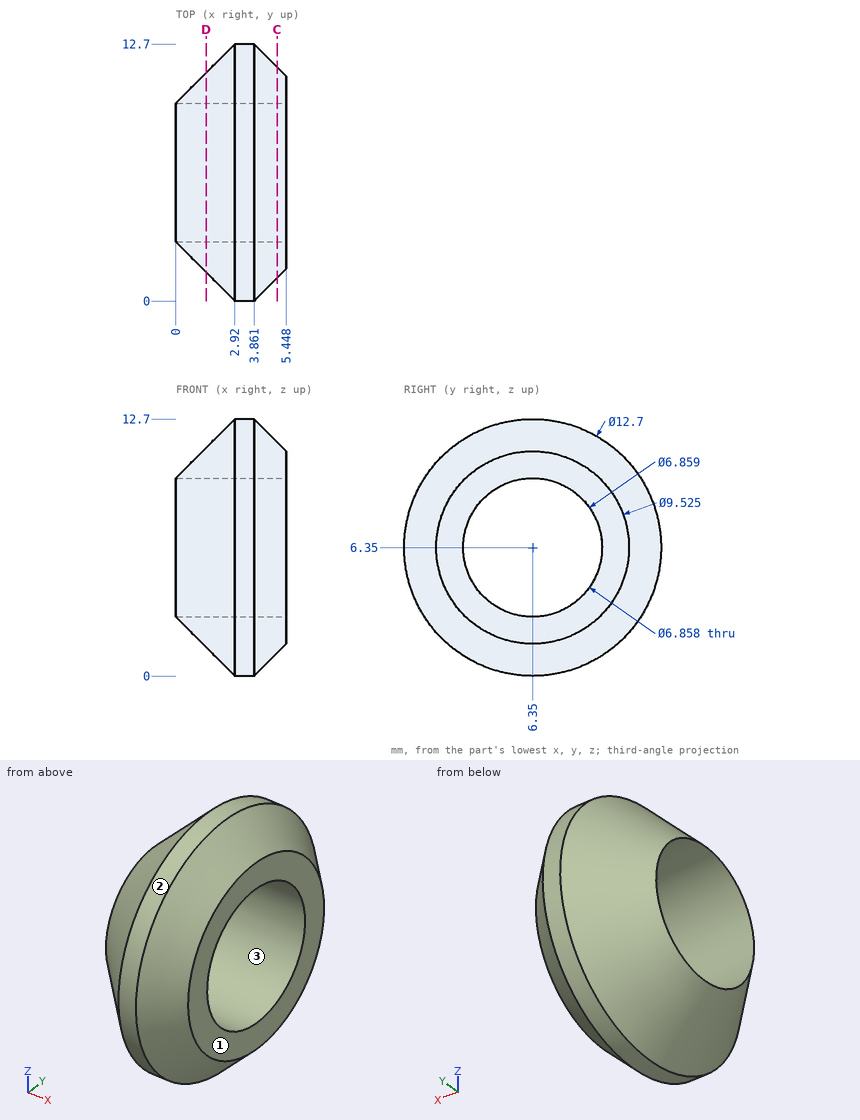
Answer from the drawing. Dimensions are ordinates in mm from the lowest x, y and z of the part. Give positions to 0.01 mm unless a question says otherwise; leave off trailing zeros. Loops run counter-clockwise (first coordinate to the right, second up) from the corner with the lowest first, then second, coordinate; pieces in that order, holes last.
Item 1: The part is cut by section D-D (x = 1.5). Write down the section's boundary in (y, z).
Item 2: Each of these flat-tipped pins is pushed along its axis until it touches: pin 1 Ø1.5 at (x, y) = (1, 2) entering from -Z (1 decimal); pin 2 Ø3 at (x, z) = (2.5, 10.5) entering from -Y; pin 3 Ø1.5 at (y, z) = (8.5, 2.5) entering from -X. Where does it stop, or does it pass through?
Item 3: The part is cut by section C-C (x = 5). Write down the section's boundary in (y, z).
Item 4: Find the intervals of material crossed by line 1 along Z through (x, y) = (3.45, 6.35); line 2 along Y through (x, z) = (2.2, 4.5) (1 decimal), in increasing order.
Item 5: The mould has two halves that part along Y. Classify the marked faces 1, 2 and 3: released by +Y, released by -Y, zero draft, split by the parting line, or undercut.
Taken from the geometry:
1. outline: circle Ø9.86 at (6.35, 6.35); hole circle Ø6.86 at (6.35, 6.35)
2. pin 1: stops at z = 3.2
2. pin 2: stops at y = 0.61
2. pin 3: stops at x = 0.23
3. outline: circle Ø10.42 at (6.35, 6.35); hole circle Ø6.86 at (6.35, 6.35)
4. line 1: z = 0 to 2.92, 9.78 to 12.7
4. line 2: y = 1 to 3.5, 9.2 to 11.7
5. face 1: zero draft
5. face 2: split by the parting line
5. face 3: undercut
